Read the model definition and answer for the solid it produces. Units are mm, in the model's axes. Give positions to 0.01 mm unless a question says otherwise; leave off trailing zeros. Write each loop counter-clockwise with the first axis right and the second up, starting at its lowest first coordinate (ties: lowest second). Pieces come first, ordered by that corner, then holes. Notation, with made-up numbers: M 81.25,52 L 139.25,52 A26 cw 139.25,91 Z; hole C -20.75,70 d1. An arc over 180 degrees is marked long. Put each result on its own line as item: value.
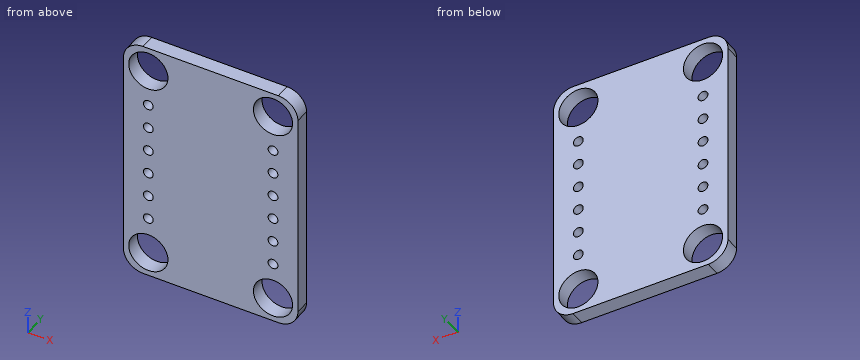
Autodesk Inventor part; units mm, degrees
ref_plane "YZ Plane" through (0, 0, 0) normal (1, 0, 0) x (0, 1, 0)
ref_plane "XZ Plane" through (0, 0, 0) normal (0, 1, 0) x (-1, 0, 0)
ref_plane "XY Plane" through (0, 0, 0) normal (0, 0, 1) x (1, 0, 0)
sketch "Szkic1" plane through (0, 0, 0) normal (0, 1, 0) x (-1, 0, 0)
  line L0 (2, 0) -> (15.8, 0)
  line L1 (17.8, -2) -> (17.8, -23.4)
  line L2 (15.8, -25.4) -> (2, -25.4)
  line L3 (0, -23.4) -> (0, -2)
  arc A0 (17.8, -2) -> (15.8, 0) centre (15.8, -2) ccw
  arc A1 (15.8, -25.4) -> (17.8, -23.4) centre (15.8, -23.4) ccw
  arc A2 (0, -23.4) -> (2, -25.4) centre (2, -23.4) ccw
  arc A3 (2, 0) -> (0, -2) centre (2, -2) ccw
  point P0 (0, 0)
  point P1 (17.8, -25.4)
  point P2 (17.8, 0)
  point P3 (0, -25.4)
  dimension "d0" = 17.8
  dimension "d1" = 25.4
  dimension "d2" = 2
extrude "Wyciągnięcie proste1" add sketch "Szkic1" along normal blind 1.5
sketch "Szkic2" plane through (0, 1.5, 0) normal (0, 1, 0) x (1, 0, 0)
  line L0 (-2, 25.4) -> (-15.8, 25.4)
  line L1 (-17.8, 23.4) -> (-17.8, 2)
  line L2 (0, 2) -> (0, 23.4)
  point P0 (0, 0)
  point P1 (-2.54, 6.35)
  point P2 (-2.54, 8.89)
  point P3 (-2.54, 11.43)
  point P4 (-2.54, 13.97)
  point P5 (-15.26, 6.35)
  point P6 (-15.26, 8.89)
  point P7 (-15.26, 11.43)
  point P8 (-15.26, 13.97)
  point P9 (-15.26, 16.51)
  point P10 (-15.26, 19.05)
  point P11 (-2.54, 16.51)
  point P12 (-2.54, 19.05)
  dimension "d8" = 2.54
  dimension "d9" = 2.54
  dimension "d10" = 2.54
  dimension "d11" = 2.54
  dimension "d12" = 2.54
  dimension "d13" = 6.35
  dimension "d14" = 2.54
  dimension "d15" = 2.54
  dimension "d16" = 2.54
  dimension "d17" = 2.54
  dimension "d19" = 2.54
hole "Otwór1" at (-2.54, 1.5, -6.35) at (-2.54, 1.5, -8.89) at (-2.54, 1.5, -11.43) at (-2.54, 1.5, -13.97) at (-15.26, 1.5, -6.35) at (-15.26, 1.5, -8.89) at (-15.26, 1.5, -11.43) at (-15.26, 1.5, -13.97) at (-15.26, 1.5, -16.51) at (-15.26, 1.5, -19.05) at (-2.54, 1.5, -16.51) at (-2.54, 1.5, -19.05) direction (0, -1, 0) diameter 1 end through all
sketch "Szkic3" plane through (0, 1.5, 0) normal (0, 1, 0) x (1, 0, 0)
  point P0 (0, 0)
sketch "Szkic4" plane through (0, 1.5, 0) normal (0, 1, 0) x (1, 0, 0)
  circle A0 centre (-2.54, 13.97) radius 0.5 construction
  circle A1 centre (-2.54, 7.62) radius 0.5 construction
  line L0 (-2.54, 13.97) -> (-2.54, 7.62) construction
  line L1 (-2.54, 13.97) -> (-2.54, -5.3346) construction
  circle A2 centre (-2.54, 8.89) radius 0.5 construction
  line L2 (-2.54, 8.89) -> (-2.54, 22.9895) construction
  circle A3 centre (-2.54, 22.86) radius 2
  line L3 (-2, 25.4) -> (-15.8, 25.4)
  circle A4 centre (-2.54, 2.54) radius 2
  line L4 (-15.8, 0) -> (-2, 0)
  circle A5 centre (-15.26, 2.54) radius 2
  circle A6 centre (-15.26, 22.86) radius 2
  line L5 (-17.8, 23.4) -> (-17.8, 2)
  point P0 (0, 0)
  dimension "d27" = 4
  dimension "d28" = 2.54
  dimension "d29" = 4
  dimension "d30" = 2.54
  dimension "d33" = 4
  dimension "d34" = 4
  dimension "d35" = 2.54
extrude "Wyciągnięcie proste2" cut sketch "Szkic4" against normal blind 10
equation "\"d6\" = d5"
equation "\"d7\" = d6"
properties part number "Adafruit_IMU"
(1) Section A-A on z = -19.05 is taken. Determine the outline of the cut face in (x, y), and give its area (3 significant figures).
Result:
outline: M -17.8,0 L -15.76,0 L -15.76,1.5 L -17.8,1.5 Z; M -14.76,0 L -3.04,0 L -3.04,1.5 L -14.76,1.5 Z; M -2.04,0 L 0,0 L 0,1.5 L -2.04,1.5 Z
area: 23.7 mm²
(2) Section B-B on x = -1.75 is taken. Determine the outline of the cut face in (y, z).
Result:
outline: M 0,-25.38 L 1.5,-25.38 L 1.5,-24.7 L 0,-24.7 Z; M 0,-21.02 L 1.5,-21.02 L 1.5,-4.38 L 0,-4.38 Z; M 0,-0.7 L 1.5,-0.7 L 1.5,-0.02 L 0,-0.02 Z
(3) Straight lines are drawn through the part: line 1 along X through (y, z) = (0.5, -19); line 2 along X through (y, z) = (0.9, -6.5); line 3 along Z through (x, y) = (-14, 0.35). For each, find the intervals that lie inside material, in ascending order. Write a range as from..to.
Result:
line 1: x = -17.8..-15.76, -14.76..-3.04, -2.04..0
line 2: x = -17.8..-15.74, -14.78..-3.02, -2.06..0
line 3: z = -25.4..-24.41, -21.31..-4.09, -0.99..0
(4) Given pin 1 Ø3.5 at (x, z) = (-2.54, -22.86) entering from -Y, flat-ended and moving along its own axis, determine where the tip first touches the part or whether it passes through.
Result:
pin 1: passes through
(5) Section C-C on y = 0.4 is taken. Give the number of separate pieces and of enclosed holes in the cut face, and give its area (3 significant figures).
Result:
separate pieces: 1
enclosed holes: 16
area: 389 mm²
